```python
from build123d import *

# Parameters (mm, degrees)
SKETCH1_W               = 50
SKETCH1_H               = 24
SKETCH1_R               = 8.25
BOSS_EXTRUDE1_DEPTH     = 7
SKETCH2_W               = 12.5
SKETCH2_H               = 4.5
CUT_EXTRUDE1_DEPTH      = 4.022504106
SKETCH3_W               = 50
SKETCH3_H               = 16
SKETCH3_R               = 1.55
BOSS_EXTRUDE2_DEPTH     = 2
CUT_EXTRUDE2_DEPTH      = 25
CUT_EXTRUDE2_DEPTH_BACK = 3
FILLET1_R               = 5
FILLET2_R               = 2
SKETCH5_W               = 57.1125727
SKETCH5_H               = 23.157416517
CUT_EXTRUDE3_DEPTH      = 1
SKETCH6_W               = 10
SKETCH6_H               = 4
CUT_EXTRUDE4_DEPTH      = 2
FILLET3_R               = 1
FILLET4_R               = 2


with BuildPart() as part:
    # Sketch1 → Boss-Extrude1 (new body)
    with BuildSketch(Plane(origin=(0, 0, 0), x_dir=(1, 0, 0), z_dir=(0, 1, 0))):
        with Locations((-25, 12)):
            Rectangle(SKETCH1_W, SKETCH1_H)
        with Locations((-38.25, 12)):
            Circle(SKETCH1_R, mode=Mode.SUBTRACT)
        with Locations((-11.75, 12)):
            Circle(SKETCH1_R, mode=Mode.SUBTRACT)
    extrude(amount=BOSS_EXTRUDE1_DEPTH)

    # Sketch2 → Cut-Extrude1 (cut)
    with BuildSketch(Plane.XZ):
        with Locations((-25, -19.75)):
            Rectangle(SKETCH2_W, SKETCH2_H)
    extrude(amount=-CUT_EXTRUDE1_DEPTH, mode=Mode.SUBTRACT)

    # Sketch3 → Boss-Extrude2 (add)
    with BuildSketch(Plane(origin=(0, 0, -24), x_dir=(-1, 0, 0), z_dir=(0, 0, -1))):
        with Locations((25, -1)):
            Rectangle(SKETCH3_W, SKETCH3_H)
        with Locations((12.5, -6)):
            Circle(SKETCH3_R, mode=Mode.SUBTRACT)
        with Locations((37.5, -6)):
            Circle(SKETCH3_R, mode=Mode.SUBTRACT)
    extrude(amount=BOSS_EXTRUDE2_DEPTH)

    # Sketch4 → Cut-Extrude2 (cut, two sides)
    with BuildSketch(Plane.XY.offset(-24)) as cut_extrude2_sk:
        Polygon((-50, 7), (-45, -9), (-50, -9), align=None)
        Polygon((0, 7), (0, -9), (-5, -9), align=None)
    extrude(amount=CUT_EXTRUDE2_DEPTH, mode=Mode.SUBTRACT)
    extrude(cut_extrude2_sk.sketch, amount=-CUT_EXTRUDE2_DEPTH_BACK, mode=Mode.SUBTRACT)

    # Fillet1
    fillet1_edges = [part.edges().sort_by_distance(p)[0] for p in [
        (-45, -9, -25),
        (-5, -9, -25),
    ]]
    fillet(fillet1_edges, radius=FILLET1_R)

    # Fillet2
    fillet2_edges = [part.edges().sort_by_distance(p)[0] for p in [
        (0, 7, -13),
        (-50, 7, -13),
    ]]
    fillet(fillet2_edges, radius=FILLET2_R)

    # Sketch5 → Cut-Extrude3 (cut)
    with BuildSketch(Plane.XY):
        with Locations((-24.983022422, 0.513257307)):
            Rectangle(SKETCH5_W, SKETCH5_H)
    extrude(amount=-CUT_EXTRUDE3_DEPTH, mode=Mode.SUBTRACT)

    # Sketch6 → Cut-Extrude4 (cut)
    with BuildSketch(Plane.XZ):
        with Locations((-25, -3)):
            Rectangle(SKETCH6_W, SKETCH6_H)
    extrude(amount=-CUT_EXTRUDE4_DEPTH, mode=Mode.SUBTRACT)

    # Fillet3
    fillet3_edges = [part.edges().sort_by_distance(p)[0] for p in [
        (-30, 1, -5),
        (-20, 1, -5),
    ]]
    fillet(fillet3_edges, radius=FILLET3_R)

    # Fillet4
    fillet4_edges = [part.edges().sort_by_distance(p)[0] for p in [
        (-30, 1, -1),
        (-20, 1, -1),
    ]]
    fillet(fillet4_edges, radius=FILLET4_R)


solid = part.part
```
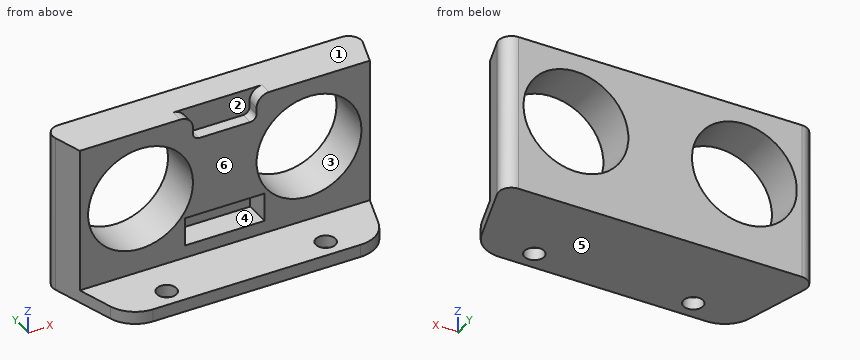
Here's how the part is built. I have some questions about the finished solid (model axes, mm). Face numbers are marked on the shaded views. A direction names the side the tool comes from. Give positions to 0.01 mm unless a question says otherwise; leave off trailing zeros. Loops run counter-clockwise (first coordinate to the right, second up) from the corner with the lowest first, then second, coordinate; pieces in that order, holes last. Notation, with made-up numbers: M 14.5,21 L 25.5,21 A9 ccw 25.5,38 Z; hole C 16,47 d6. An arc over 180 degrees is marked long. Put each result on its own line as item: value. Start each with the question number.
(1) I want a section at C-C on y = 1. Please give me the cut outline in (x, z) (3 decimals).
(2) I want a section at B-B on x = -11.75. Please give me the cut outline in (y, z).
(3) I want a section at A-A on z = -12. Please give me the cut outline in (x, y), then the cut area to 3 significant figures.
(4) For the marked faces 4, 5 and 6, which set-ups out of +Z, -Z, +X, -X, +Y, -Y let a thin tool reach every point of the face, with its end or its side?
(5) Will these pins go through, and if not, where does the flat tip stop? pin 1 Ø3.5 at (x, y) = (-37.5, -6) entering from +Z; pin 2 Ø1.2 at (y, z) = (3, -19.5) entering from -X; pin 3 Ø3 at (x, z) = (-26, -3) entering from -Y.
(6) I need wall thicknesses on line 1 along X through (y, z) = (4, -15.5); line 2 along Z through (x, y) = (-38.25, 3.5); line 3 along X through (y, z) = (0.5, -15.75). Which ranges of each line are inside material? Lowest first, please. Write a range as [from, to].
(7) I want a section at D-D on y = -6. Please give me the cut outline in (x, z).
(8) If we mould it in two halves opening along Z, with no side actions, what happens to the marked faces 1, 2 and 3? For each: +Z half, -Z half, draft (parallel to the pull), parting line (faces both ways), or undercut.
Answer block:
1. outline: M -48.125,-26 L -1.875,-26 L -1.875,-1 L -18,-1 A2 ccw -20,-3 L -20,-4 A1 cw -21,-5 L -29,-5 A1 cw -30,-4 L -30,-3 A2 ccw -32,-1 L -48.125,-1 Z; hole C -38.25,-12 d16.5; hole M -31.25,-22 L -18.75,-22 L -18.75,-17.5 L -31.25,-17.5 Z; hole C -11.75,-12 d16.5
2. outline: M -9,-26 L -7.36,-26 L -7.36,-24 L -9,-24 Z; M -4.64,-26 L 7,-26 L 7,-20.25 L 0,-20.25 L 0,-24 L -4.64,-24 Z; M 0,-3.75 L 7,-3.75 L 7,-1 L 0,-1 Z
3. outline: M -49.19,4.4 L -47.81,0 L -46.5,0 L -46.5,7 L -47.28,7 A2 ccw Z; M -30,0 L -20,0 L -20,7 L -30,7 Z; M -3.5,0 L -2.19,0 L -0.81,4.4 A2 ccw -2.72,7 L -3.5,7 Z
3. area: 100 mm^2
4. face 4: -Y
4. face 5: -Z, +X, -X, +Y, -Y
4. face 6: +Z, +X, -X, -Y
5. pin 1: z = -24
5. pin 2: x = -48.94
5. pin 3: y = 2
6. line 1: [-49.06, -45.72], [-30.78, -19.22], [-4.28, -0.94]
6. line 2: [-26, -20.25], [-3.75, -1]
6. line 3: [-47.97, -45.6], [-30.9, -19.1], [-4.4, -2.03]
7. outline: M -45.91,-26 L -39.05,-26 L -39.05,-24 L -45.91,-24 Z; M -35.95,-26 L -14.05,-26 L -14.05,-24 L -35.95,-24 Z; M -10.95,-26 L -4.09,-26 L -4.09,-24 L -10.95,-24 Z
8. face 1: +Z half
8. face 2: draft
8. face 3: undercut
